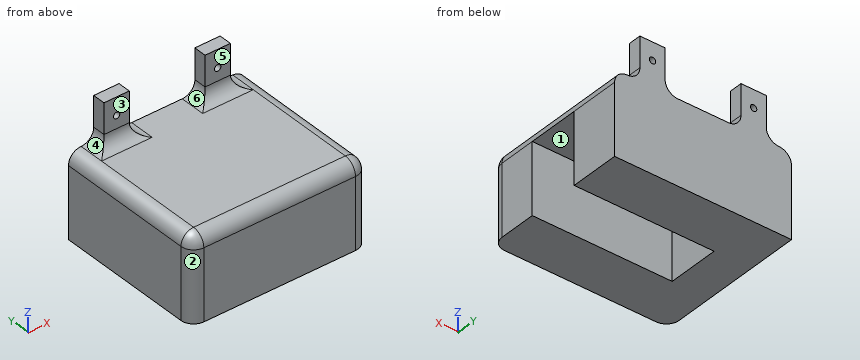
```python
from build123d import *

# Parameters (mm, degrees)
SKETCH_2_W          = 70
SKETCH_2_H          = 60
EXTRUDE_2_DEPTH     = 33
SKETCH_3_W          = 40.7
SKETCH_3_H          = 20.5
CUT_EXTRUDE_1_DEPTH = 28
SKETCH_4_W          = 14.65
SKETCH_4_H          = 20.5
EXTRUDE_3_DEPTH     = 28
SKETCH_5_W          = 14.65
SKETCH_5_H          = 20.5
CUT_EXTRUDE_4_DEPTH = 28
SKETCH_8_W          = 10
SKETCH_8_H          = 5
EXTRUDE_5_DEPTH     = 50
M3X0_5_1_D          = 2.5
FILLET_1_R          = 5
FILLET_2_R          = 5
FILLET_3_R          = 5


# Some blends are built 0.0001 mm under size
with BuildPart() as part:
    # ｽｹｯﾁ2 → ﾎﾞｽ - 押し出し2 (new body)
    with BuildSketch(Plane.XY):
        Rectangle(SKETCH_2_W, SKETCH_2_H)
    extrude(amount=EXTRUDE_2_DEPTH)

    # ｽｹｯﾁ3 → ｶｯﾄ - 押し出し1 (cut)
    with BuildSketch(Plane.XY):
        Rectangle(SKETCH_3_W, SKETCH_3_H)
    extrude(amount=CUT_EXTRUDE_1_DEPTH, mode=Mode.SUBTRACT)

    # ｽｹｯﾁ4 → ﾎﾞｽ - 押し出し3 (add)
    with BuildSketch(Plane.XY):
        with Locations((27.675, 0)):
            Rectangle(SKETCH_4_W, SKETCH_4_H)
    extrude(amount=EXTRUDE_3_DEPTH)

    # ｽｹｯﾁ5 → ｶｯﾄ - 押し出し4 (cut)
    with BuildSketch(Plane.XY):
        with Locations((27.675, 0)):
            Rectangle(SKETCH_5_W, SKETCH_5_H)
    extrude(amount=CUT_EXTRUDE_4_DEPTH, mode=Mode.SUBTRACT)

    # ｽｹｯﾁ8 → ﾎﾞｽ - 押し出し5 (add)
    with BuildSketch(Plane.XY):
        with Locations((-20, 27.5)):
            Rectangle(SKETCH_8_W, SKETCH_8_H)
        with Locations((20, 27.5)):
            Rectangle(SKETCH_8_W, SKETCH_8_H)
    extrude(amount=EXTRUDE_5_DEPTH)

    # M3x0.5 ねじ穴1 (through all)
    with Locations(Plane(origin=(0, 30, 0), x_dir=(1, 0, 0), z_dir=(0, 1, 0))):
        with Locations((-20, -43), (20, -43)):
            Hole(M3X0_5_1_D / 2)

    # ﾌｨﾚｯﾄ1
    fillet_1_edges = [part.edges().sort_by_distance(p)[0] for p in [
        (-15, 27.5, 33),
        (-20, 25, 33),
        (-25, 27.5, 33),
        (20, 25, 33),
        (15, 27.5, 33),
        (25, 27.5, 33),
    ]]
    fillet(fillet_1_edges, radius=FILLET_1_R)

    # ﾌｨﾚｯﾄ2
    fillet_2_edges = [part.edges().sort_by_distance(p)[0] for p in [
        (35, 0, 33),
        (35, -30, 16.5),
        (0, -30, 33),
        (-35, 0, 33),
    ]]
    fillet(fillet_2_edges, radius=FILLET_2_R - 0.0001)  # a hair under: the kernel refuses the full size

    # ﾌｨﾚｯﾄ3
    # the kernel refuses this fillet: 5 mm, written as the material it takes off along each edge
    with BuildSketch(Plane(origin=(-30, -25, 33), x_dir=(-1, 0, 0), z_dir=(0, 1, 0))) as fillet_3_piece_1:
        with BuildLine():
            CenterArc((0.0001, -4.9999), 4.9999, 0, 90)
            Line((5, -4.9999), (5, 0))
            Line((5, 0), (0.0001, 0))
        make_face()
    revolve(axis=Axis((-30, -25, 33), (0, 0, 1)), revolution_arc=90, mode=Mode.SUBTRACT)
    with BuildSketch(Plane(origin=(-35, -30, -12.5), x_dir=(0, 1, 0), z_dir=(0, 0, 1))) as fillet_3_piece_2:
        with BuildLine():
            CenterArc((FILLET_3_R, -FILLET_3_R), FILLET_3_R, 90, 90)
            Line((0, -FILLET_3_R), (0, 0))
            Line((0, 0), (FILLET_3_R, 0))
        make_face()
    extrude(amount=45.5, mode=Mode.SUBTRACT)


solid = part.part
```
CAD build for the part. Positions are in the model's coordinates, mm. Face numbers are marked on the shaded views. A direction names the side the tool comes from. Coordinates: 2 decimals unless noted, no trailing zeros. Write each loop counter-clockwise with the first axis right and the second up, starting at its lowest first coordinate (ties: lowest second). Pieces come first, ordered by that corner, then holes.
(1) Drill centre lines: probe 1 along X at (y, z) = (28, 43); probe 2 along Y at (x, z) = (16, 21); probe 3 along Z at (x, y) = (-20, 26.5). Where is each one in solid material? Low to high.
(2) 3-axis set-ups, long thin cutter, end or side, ignore diameter. For the marked faces 1, 2 and 3: which of +Z, -Z, +X, -X, +Y, -Y reach the whole face in a straight line?
(3) Flat gauge pins, fed straight in: pin 1 (8 mm diameter, centred on y = -23.5, z = 36.5, fed in from +X); pin 2 (8 mm diameter, centred on x = -20, z = 41, fed in from -Y); pin 3 (4 mm diameter, centred on y = 27, z = 46.5, fed in from +X). Where does each tip first touch, or does it go through?
(4) Cut at D-D, the plane x = 7. List the corners of the cut face in (y, z).
(5) Cut at A-A, the plane x = 20. List the corners of the cut face in (y, z).
(6) Two-plate mould, pull along X, no slides. Class the marked faces 4, 5 and 6: +X half, -X half, draft (parallel to the pull), parting line (faces both ways), or undercut.
(7) Cut at B-B, the plane z = 43. List the corners of the cut face in (x, y).
Geometry says:
1. probe 1: x = -25 to -21.25, -18.75 to -15, 15 to 18.75, 21.25 to 25
1. probe 2: y = -30 to -10.25, 10.25 to 30
1. probe 3: z = 0 to 41.75, 44.25 to 50
2. face 1: -Z, +X
2. face 2: +Z, -Z, -X, -Y
2. face 3: +Z, +X, -X, -Y
3. pin 1: stops at x = 32.18
3. pin 2: stops at y = 24.9
3. pin 3: stops at x = 25
4. outline: (-30, 0) - (-10.25, 0) - (-10.25, 28) - (10.25, 28) - (10.25, 0) - (30, 0) - (30, 33) - (-25, 33) arc R5 ccw to (-30, 28) - close
5. outline: (-30, 0) - (-10.25, 0) - (-10.25, 28) - (10.25, 28) - (10.25, 0) - (30, 0) - (30, 41.75) - (25, 41.75) - (25, 38) arc R5 cw to (20, 33) - (-25, 33) arc R5 ccw to (-30, 28) - close; (25, 44.25) - (30, 44.25) - (30, 50) - (25, 50) - close
6. face 4: -X half
6. face 5: draft
6. face 6: undercut
7. outline: (-25, 25) - (-21.25, 25) - (-21.25, 30) - (-25, 30) - close; (-18.75, 25) - (-15, 25) - (-15, 30) - (-18.75, 30) - close; (15, 25) - (18.75, 25) - (18.75, 30) - (15, 30) - close; (21.25, 25) - (25, 25) - (25, 30) - (21.25, 30) - close
